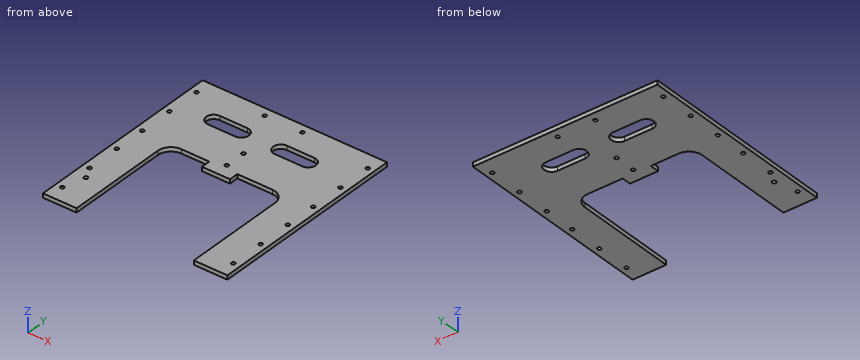
Autodesk Inventor part; units mm, degrees
ref_plane "YZ Plane" through (0, 0, 0) normal (1, 0, 0) x (0, 1, 0)
ref_plane "XZ Plane" through (0, 0, 0) normal (0, 1, 0) x (-1, 0, 0)
ref_plane "XY Plane" through (0, 0, 0) normal (0, 0, 1) x (1, 0, 0)
sketch "Sketch1" plane through (0, 0, 0) normal (0, 0, 1) x (1, 0, 0)
  circle A0 centre (-10.075, 23.3762) radius 2.8
  circle A1 centre (-10.075, -28.6238) radius 2.8
  circle A2 centre (-10.075, -80.6238) radius 2.8
  circle A3 centre (-10.075, -129.3175) radius 2.8
  circle A4 centre (-10.075, -181.3175) radius 2.8
  circle A5 centre (-10.075, -233.3175) radius 2.8
  circle A6 centre (-269.521, -233.3175) radius 2.8
  circle A7 centre (-269.521, -181.3175) radius 2.8
  circle A8 centre (-269.521, -129.3175) radius 2.8
  circle A9 centre (-269.521, -80.6238) radius 2.8
  circle A10 centre (-269.521, -28.6238) radius 2.8
  circle A11 centre (-269.521, 23.3762) radius 2.8
  line L0 (-279.596, -257.6643) -> (-279.596, 47.723)
  line L1 (0, 47.723) -> (0, -257.6643)
  line L2 (-50.898, -102.277) -> (-50.898, -257.6643)
  line L3 (-228.698, -257.6643) -> (-228.698, -102.277)
  line L4 (0, 47.723) -> (-279.596, 47.723)
  line L5 (-279.596, -257.6643) -> (-228.698, -257.6643)
  line L6 (-50.898, -257.6643) -> (0, -257.6643)
  circle A12 centre (-145.1723, -43.7167) radius 2.8
  circle A13 centre (-175.2462, 34.723) radius 2.75
  circle A14 centre (-118.0962, 34.723) radius 2.75
  circle A15 centre (-260.35, -200.025) radius 3
  line L7 (-123.9223, -92.277) -> (-123.9223, -96.277)
  line L8 (-166.4223, -96.277) -> (-166.4223, -92.277)
  circle A16 centre (-145.1723, -75.7167) radius 2.8
  line L9 (-145.1723, -75.7167) -> (-145.1723, -72.9167) construction
  line L10 (-145.1723, -46.5167) -> (-145.1723, 47.723) construction
  line L11 (-123.9223, -82.277) -> (-123.9223, -92.277)
  line L12 (-166.4223, -82.277) -> (-166.4223, -92.277)
  line L13 (-70.898, -82.277) -> (-123.9223, -82.277)
  line L14 (-166.4223, -82.277) -> (-208.698, -82.277)
  line L15 (-123.9223, -96.277) -> (-166.4223, -96.277)
  line L16 (-73.5425, -10.0701) -> (-115.2306, -10.0701) construction
  line L17 (-73.5425, 1.3522) -> (-115.2306, 1.3522)
  line L18 (-115.2306, -21.4924) -> (-73.5425, -21.4924)
  arc A17 (-73.5425, -21.4924) -> (-73.5425, 1.3522) centre (-73.5425, -10.0701) ccw
  arc A18 (-115.2306, 1.3522) -> (-115.2306, -21.4924) centre (-115.2306, -10.0701) ccw
  line L19 (-216.8021, -10.0701) -> (-175.1139, -10.0701) construction
  line L20 (-216.8021, 1.3522) -> (-175.1139, 1.3522)
  line L21 (-175.1139, -21.4924) -> (-216.8021, -21.4924)
  arc A19 (-216.8021, 1.3522) -> (-216.8021, -21.4924) centre (-216.8021, -10.0701) ccw
  arc A20 (-175.1139, -21.4924) -> (-175.1139, 1.3522) centre (-175.1139, -10.0701) ccw
  arc A21 (-50.898, -102.277) -> (-70.898, -82.277) centre (-70.898, -102.277) ccw
  arc A22 (-208.698, -82.277) -> (-228.698, -102.277) centre (-208.698, -102.277) ccw
  point P0 (-50.898, -82.277)
  point P1 (-228.698, -82.277)
  point P2 (-94.3865, -10.0701)
  point P3 (-195.958, -10.0701)
  dimension "d12" = 5.6
  dimension "d13" = 5.6
  dimension "d2" = 305.3873
  dimension "d3" = 279.596
  dimension "d7" = 5.5
  dimension "d14" = 32
  dimension "d16" = 94.2398
  dimension "d22" = 20
extrude "Extrusion1" add sketch "Sketch1" along normal blind 6.35
properties part number "Mech Chassis v7 deckipt" material "Polycarbonate, Clear"
Here's how the part is built. I have some questions about the finished solid (model axes, mm). Round coordinates to 2 decimals unless told otherwise and drop trailing zeros. Order: outer loops, then holes, each group sorted by start corner. A loop starts at its lowest first (then second) coordinate and runs counter-clockwise, first axis right, second up. Notation, with made-up numbers: (19.5, 46) -> (50.5, 46) arc R20 cw to (50.5, 66) -> close; hole circle Ø3 at (-23, -37). An arc over 180 degrees is marked (long way). Use a Markdown table: item, result. Add a question column.
(1) I need wall thicknesses on line 1 along X through (y, z) = (-10, 5); line 2 along Y through (x, z) = (-177, 2.25); line 3 along X through (y, z) = (-125.5, 3.25). Which ranges of each line are inside material? Lowest first, please.
(2) Suppose I cut it at B-B, the plane z = 3.25. Count the separate pieces of the cut face and the enclosed holes in it, and give its area (3 significant figures).
(3) Suppose I cut it at A-A, the plane y = -147. Please give me the cut outline in (x, z), and give its area (3 significant figures).
(4) For pin 1 Ø7.5 at (x, y) = (-10.07, -80.62) entering from -Z, with a flat end and sliding along its axis, tell me the tip position at first contact or that it passes through.
Verdict:
| question | item | result |
|---|---|---|
| 1 | line 1 | -279.6 to -228.22, -163.69 to -126.65, -62.12 to 0 |
| 1 | line 2 | -82.28 to -21.49, 1.35 to 32.6, 36.84 to 47.72 |
| 1 | line 3 | -279.6 to -228.7, -50.9 to 0 |
| 2 | separate pieces | 1 |
| 2 | enclosed holes | 19 |
| 2 | area | 51,800 mm2 |
| 3 | outline | (-279.6, 0) -> (-228.7, 0) -> (-228.7, 6.35) -> (-279.6, 6.35) -> close; (-50.9, 0) -> (0, 0) -> (0, 6.35) -> (-50.9, 6.35) -> close |
| 3 | area | 646 mm2 |
| 4 | pin 1 | z = 0 |
